from build123d import *

# Parameters (mm, degrees)
SKETCH1_W           = 40.5
SKETCH1_H           = 2.7
BOSS_EXTRUDE1_DEPTH = 2.7


with BuildPart() as part:
    # Sketch1 → Boss-Extrude1 (new body)
    with BuildSketch(Plane(origin=(0, 0, 0), x_dir=(1, 0, 0), z_dir=(0, 1, 0))):
        Polygon((-60.75, 13.3), (-20.25, 13.3), (-20.25, 10.6), (20.25, 10.6), (20.25, 13.3), (60.75, 13.3), (60.75, -13.3), (36.45, -13.3), (36.45, -8.3), (12.15, -8.3), (12.15, -13.3), (-12.15, -13.3), (-12.15, -8.3), (-36.45, -8.3), (-36.45, -13.3), (-60.75, -13.3), align=None)
        with Locations((0, -1.95)):
            Rectangle(SKETCH1_W, SKETCH1_H, mode=Mode.SUBTRACT)
    extrude(amount=BOSS_EXTRUDE1_DEPTH)


solid = part.part
Can you work these out from the model? Positions are in its coordinate system, mm. A direction names the side the tool comes from. Give positions to 0.01 mm unless a question says otherwise; leave off trailing zeros. Write each loop counter-clockwise with the first axis right and the second up, starting at its lowest first coordinate (ties: lowest second). Pieces come first, ordered by that corner, then holes. Notation, with made-up numbers: (16, 24.5) -> (35, 24.5) arc R15 ccw to (35, 50.5) -> close; hole circle Ø6 at (-28, 26). An arc over 180 degrees is marked (long way). Answer as a JSON object with one key per item and string values. Group by question number.
Item 1: Suppose I cut it at D-D (x = 34.5). Please give me the cut outline in (y, z), plus the area to 3 significant figures.
Item 2: Suppose I cut it at A-A (y = 0.85). Please give me the cut outline in (x, z).
Item 3: We'd pull the mould along X, two halves only. Please class faces 1 (the face through (-60.75, 1, 0)), 2 (the face through (40, 1, -13.3)), 3 (the face through (0, 1, -10.6)): +X half, -X half, draft (parallel to the pull), parting line (faces both ways), or undercut.
Item 4: Suppose I cut it at C-C (z = 10). Please give me the cut outline in (x, y), plus the area to 3 significant figures.
Item 5: For faces 4 (the face through (-20.25, 1, 2)), 5 (the face through (24, 1, 8.3)), 6 (the face through (20.25, 1, -12)), which set-ups out of +Z, -Z, +X, -X, +Y, -Y let a thin tool reach every point of the face, with its end or its side?
Item 6: Please list where these lines run through material, in increasing order: line 1 (X direction, y = 1.05, z = 11.5); line 2 (X direction, y = 2.3, z = -11.75); line 3 (Z direction, x = 1.5, y = 2). Write a range as [from, to].
Item 7: Suppose I cut it at B-B (x = 14.5). Please give me the cut outline in (y, z), plus the area to 3 significant figures.
Item 8: I'm going to push a flat-ended pin straight in: P1, Ø1.4, axis at x = 20.5, y = 1.5, coming from the +Z side. Where does the tip first touch, or does it pass through?
Findings:
{
 "1": {"outline": "(0, -13.3) -> (2.7, -13.3) -> (2.7, 8.3) -> (0, 8.3) -> close", "area": "58.3 mm²"},
 "2": {"outline": "(-60.75, -13.3) -> (-20.25, -13.3) -> (-20.25, -10.6) -> (20.25, -10.6) -> (20.25, -13.3) -> (60.75, -13.3) -> (60.75, 13.3) -> (36.45, 13.3) -> (36.45, 8.3) -> (12.15, 8.3) -> (12.15, 13.3) -> (-12.15, 13.3) -> (-12.15, 8.3) -> (-36.45, 8.3) -> (-36.45, 13.3) -> (-60.75, 13.3) -> close; hole (-20.25, 0.6) -> (20.25, 0.6) -> (20.25, 3.3) -> (-20.25, 3.3) -> close"},
 "3": {"face 1": "-X half", "face 2": "draft", "face 3": "undercut"},
 "4": {"outline": "(-60.75, 0) -> (-36.45, 0) -> (-36.45, 2.7) -> (-60.75, 2.7) -> close; (-12.15, 0) -> (12.15, 0) -> (12.15, 2.7) -> (-12.15, 2.7) -> close; (36.45, 0) -> (60.75, 0) -> (60.75, 2.7) -> (36.45, 2.7) -> close", "area": "197 mm²"},
 "5": {"face 4": "+Y, -Y", "face 5": "+Z, +Y, -Y", "face 6": "-Z, +Y, -Y"},
 "6": {"line 1": "x = [-60.75, -36.45], [-12.15, 12.15], [36.45, 60.75]", "line 2": "x = [-60.75, -20.25], [20.25, 60.75]", "line 3": "z = [-10.6, 0.6], [3.3, 13.3]"},
 "7": {"outline": "(0, -10.6) -> (2.7, -10.6) -> (2.7, 0.6) -> (0, 0.6) -> close; (0, 3.3) -> (2.7, 3.3) -> (2.7, 8.3) -> (0, 8.3) -> close", "area": "43.7 mm²"},
 "8": {"P1": "stops at z = 8.3"}
}
